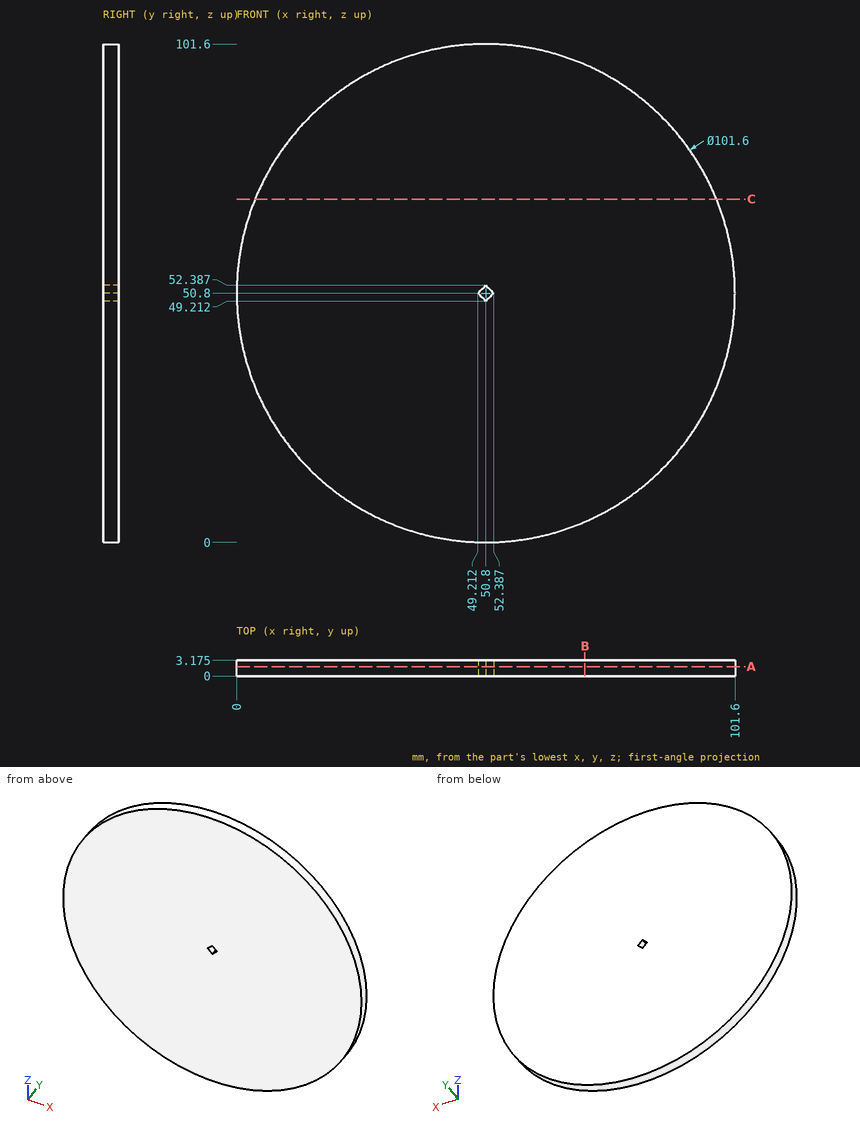
Study the drawing (mm; zero at the part's minimum x, y, z) and answer. Give positions to 0.01 mm unless a question says otherwise; leave off trailing zeros. Order: outer loops, then holes, each group sorted by start corner. A loop starts at its lowest first (then second) coordinate and runs counter-clockwise, first axis right, second up.
1) Find section A-A on y = 1.9. Write down the section's boundary in (x, z), then the cut area to 3 significant figures.
Reported:
outline: circle Ø101.6 at (50.8, 50.8); hole (49.21, 50.8) - (50.8, 49.21) - (52.39, 50.8) - (50.8, 52.39) - close
area: 8,100 mm2
2) Given P1, Ø6, axis at x = 86, z = 45, coming from the -Y side; P2, Ø1, axis at y = 2.5, z = 67.5, coming from the +X side; P3, Ø1.5, axis at x = 14, y = 0.5, coming from the -Z side, each flat-ended and moving along its own axis, determine where each tip first touches the part or whether it passes through.
Reported:
P1: stops at y = 0
P2: stops at x = 98.95
P3: stops at z = 15.01
3) Consider line 1 along Z through (x, y) = (50, 1.65) (1 decimal); line 2 along X through (y, z) = (2.65, 44); line 3 along Z through (x, y) = (22, 1.1) (1 decimal). Determine where each line is inside the solid, lowest interval first.
Reported:
line 1: z = 0 to 50, 51.6 to 101.6
line 2: x = 0.46 to 101.14
line 3: z = 9 to 92.6
4) Find section B-B on x = 71. Write down the section's boundary in (y, z) (1 decimal), then the cut area to 3 significant figures.
Reported:
outline: (0, 4.2) - (3.2, 4.2) - (3.2, 97.4) - (0, 97.4) - close
area: 296 mm2
5) Find section C-C on z = 70. Write down the section's boundary in (x, y) (1 decimal).
Reported:
outline: (3.8, 0) - (97.8, 0) - (97.8, 3.2) - (3.8, 3.2) - close
